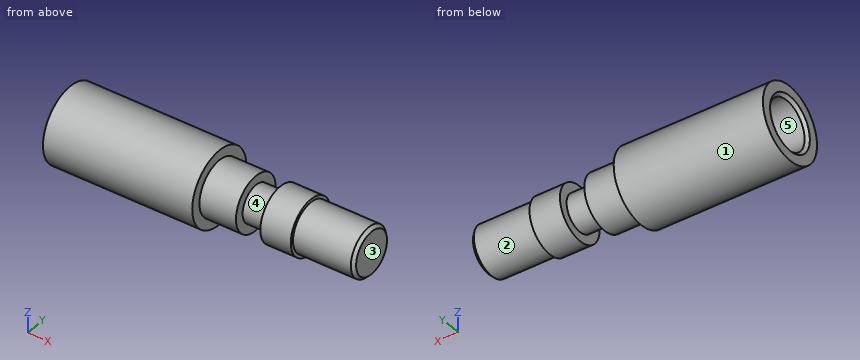
```python
from build123d import *

# Parameters (mm, degrees)
F2_SIZE = 1
F3_SIZE = 1


with BuildPart() as f1:
    # F0 (on Front) → F1 (revolve)
    with BuildSketch(Plane.XZ):
        Polygon((-49, 8), (-29, 8), (-29, 6.75), (-26, 6.75), (-26, 4.28064), (-23.732601, 0), (50, 0), (50, 8), (30, 8), (30, 9), (20, 9), (20, 6), (12, 6), (12, 9), (0, 9), (0, 12.25), (-49, 12.25), align=None)
    revolve(axis=Axis((13.1337, 0, 0), (1, 0, 0)))

    # F2
    f2_edges = [f1.edges().sort_by_distance(p)[0] for p in [
        (50, 0, -8),
    ]]
    chamfer(f2_edges, length=F2_SIZE)

    # F3
    f3_edges = [f1.edges().sort_by_distance(p)[0] for p in [
        (-49, 0, -8),
    ]]
    chamfer(f3_edges, length=F3_SIZE)


solid = f1.part
```
Geometry check sheet. Reference: the model listing, model coordinates, mm. Face numbers are marked on the shaded views. A direction names the side the tool comes from. Round coordinates to 2 decimals unless told otherwise and drop trailing zeros. Loops run counter-clockwise (first coordinate to the right, second up) from the corner with the lowest first, then second, coordinate; pieces in that order, holes last. Notation, with made-up numbers: (34.25, -28) - (69.25, -28) arc R29 cw to (69.25, -2) - close; hole circle Ø9 at (68, 6.5). An arc over 180 degrees is marked (long way). Write each question's results on one line, items separated by ' | '. Start each with the question number.
Q1. Thickness scan on line 1 (Z direction, x = -38.75, y = 0); line 2 (Y direction, x = -28.1, z = 0). Record the ranges inside material, lowest first. Write a range as [from, to].
Q2. Cross-section at B-B on x = 22.5. Enter the section's corners in (y, z), and give its area (3 significant figures).
Q3. Release check for a two-part mould opening along Y. For the marked faces 3, 4 and 5 record: +Y half, -Y half, draft (parallel to the pull), parting line (faces both ways), or undercut.
Q4. Cross-section at A-A on x = -41. Enter the section's corners in (y, z).
Q5. Access from +Z, -Z, +X, -X, +Y, -Y to the whole of each face (thin tool, end or side, straight path). Record for the marked faces 1 and 2.
Q6. Cross-section at C-C on y = 10. Enter the section's corners in (x, z).
Q7. Gauge pin test, flat ends, axial feed: P1, Ø5, axis at y = -3, z = 9.5, coming from the +X side; P2, Ø3, axis at x = 28.5, y = 6, coming from the -Z side; P3, Ø9, axis at y = 2.5, z = -0.5, coming from the -X side. Record the tip position at first contact, or that the pin passes through.
Answers below:
1) line 1: z = [-12.25, -8], [8, 12.25] | line 2: y = [-12.25, -6.75], [6.75, 12.25]
2) outline: circle Ø18 at (0, 0) | area: 254 mm²
3) face 3: draft | face 4: parting line | face 5: undercut
4) outline: circle Ø24.5 at (0, 0); hole circle Ø16 at (0, 0)
5) face 1: +X, -X | face 2: +X
6) outline: (-49, -7.08) - (0, -7.08) - (0, 7.08) - (-49, 7.08) - close
7) P1: stops at x = 49.54 | P2: stops at z = -7.79 | P3: stops at x = -29
